from build123d import *

# Parameters (mm, degrees)
SKETCH2_R           = 28.55
BOSS_EXTRUDE1_DEPTH = 12.6
SKETCH3_R           = 21
CUT_EXTRUDE1_DEPTH  = 3
SKETCH4_R           = 15.5
CUT_EXTRUDE2_DEPTH  = 24
SKETCH5_R           = 2.2
CUT_EXTRUDE3_DEPTH  = 24


with BuildPart() as part:
    # Sketch2 → Boss-Extrude1 (new body)
    with BuildSketch(Plane(origin=(0, 0, 0), x_dir=(1, 0, 0), z_dir=(0, 1, 0))):
        with Locations(Location((0, 0, 0), (0, 0, 270))):
            Circle(SKETCH2_R)
    extrude(amount=BOSS_EXTRUDE1_DEPTH)

    # Sketch3 → Cut-Extrude1 (cut)
    with BuildSketch(Plane.XZ):
        with Locations(Location((0, 0, 0), (0, 0, 270))):
            Circle(SKETCH3_R)
    extrude(amount=-CUT_EXTRUDE1_DEPTH, mode=Mode.SUBTRACT)

    # Sketch4 → Cut-Extrude2 (cut)
    with BuildSketch(Plane.XZ.offset(-3)):
        with Locations(Location((0, 0, 0), (0, 0, 270))):
            Circle(SKETCH4_R)
    extrude(amount=-CUT_EXTRUDE2_DEPTH, mode=Mode.SUBTRACT)

    # Sketch5 → Cut-Extrude3 (cut)
    with BuildSketch(Plane(origin=(0, 0, 0), x_dir=(-1, 0, 0), z_dir=(0, -1, 0))):
        with Locations(Location((-24.775, 0, 0), (0, 0, 90))):
            Circle(SKETCH5_R)
    cut_extrude3 = extrude(amount=-CUT_EXTRUDE3_DEPTH, mode=Mode.SUBTRACT)

    # Mirror1: Cut-Extrude3 across plane
    add(cut_extrude3.mirror(Plane(origin=(0, 0, 0), x_dir=(0, 0, 1), z_dir=(1, 0, 0))), mode=Mode.SUBTRACT)


solid = part.part
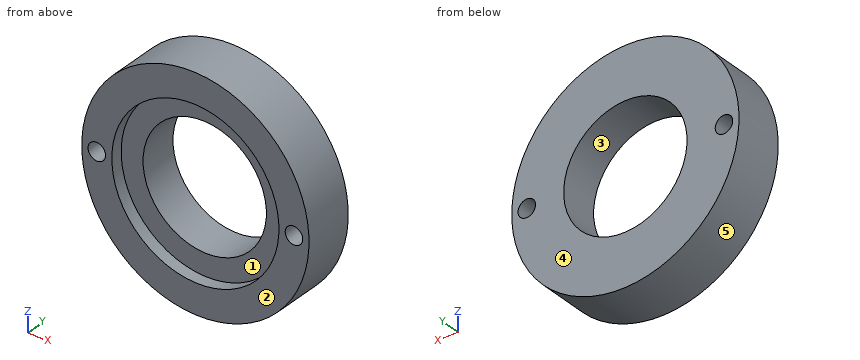
Build history of the part. All positions in model axes, mm. Face numbers are marked on the shaded views. A direction names the side the tool comes from. Coordinates: 2 decimals unless noted, no trailing zeros. Order: outer loops, then holes, each group sorted by start corner. A loop starts at its lowest first (then second) coordinate and runs counter-clockwise, first axis right, second up. Notation, with made-up numbers: (-31, 80) - (14, 80) arc R37 cw to (14, 117) - close; hole circle Ø6 at (39, 61.25). An arc over 180 degrees is marked (long way). Write item = value, one per line. Start each with the question number.
1) Two-plate mould, pull along X, no slides. Class the marked faces 3, 4 and 5: pulls with the +X half, pulls with the -X half, needs draft (parallel to the pull), parting line crosses it, or undercut.
2) Saw through at C-C on z = -14. Write the cut outline in (x, y), then the cut area to 3 significant figures.
3) Saw through at B-B on x = 0. Write the cut outline in (y, z).
4) Flat gauge pins, fed straight in: pin 1 Ø12.5 at (x, z) = (-4.5, -8) entering from -Y; pin 2 Ø1 at (y, z) = (7, -1) entering from -X; pin 3 Ø1 at (x, z) = (17, -3.5) entering from -Y; pin 4 Ø2 at (x, y) = (-13, 7.5) entering from +Z. Where does each tip first touch, or does it go through?
5) 3-axis set-ups, long thin cutter, end or side, ignore diameter. For the marked faces 1 and 2: which of +Z, -Z, +X, -X, +Y, -Y reach the whole face in a straight line?
6) Saw through at D-D on x = -18. Write the cut outline in (y, z), then the cut area to 3 significant figures.
7) Saw through at A-A on z = 0. Write the cut outline in (x, y) (3 decimals), then the cut area to 3 significant figures.
8) Wall check: line 1 along X through (y, z) = (9, 0) (3 decimals); line 2 along X through (y, z) = (1.3, 0) (3 decimals); line 3 along Z through (x, y) = (-0.5, 3.25). Give the ranges that are in metal, low to high. Write a range as from..to.
From the geometry:
q1.face_3 = undercut
q1.face_4 = needs draft
q1.face_5 = parting line crosses it
q2.outline = (-24.88, 0) - (-15.65, 0) - (-15.65, 3) - (-6.65, 3) - (-6.65, 12.6) - (-24.88, 12.6) - close; (6.65, 3) - (15.65, 3) - (15.65, 0) - (24.88, 0) - (24.88, 12.6) - (6.65, 12.6) - close
q2.area = 405 mm^2
q3.outline = (0, -28.55) - (12.6, -28.55) - (12.6, -15.5) - (3, -15.5) - (3, -21) - (0, -21) - close; (0, 21) - (3, 21) - (3, 15.5) - (12.6, 15.5) - (12.6, 28.55) - (0, 28.55) - close
q4.pin_1 = through
q4.pin_2 = -28.55
q4.pin_3 = 3
q4.pin_4 = 25.91
q5.face_1 = -Y
q5.face_2 = +Z, -Z, +X, -X, -Y
q6.outline = (0, -22.16) - (12.6, -22.16) - (12.6, 22.16) - (0, 22.16) - (0, 10.82) - (3, 10.82) - (3, -10.82) - (0, -10.82) - close
q6.area = 494 mm^2
q7.outline = (-28.55, 0) - (-26.975, 0) - (-26.975, 12.6) - (-28.55, 12.6) - close; (-22.575, 0) - (-21, 0) - (-21, 3) - (-15.5, 3) - (-15.5, 12.6) - (-22.575, 12.6) - close; (15.5, 3) - (21, 3) - (21, 0) - (22.575, 0) - (22.575, 12.6) - (15.5, 12.6) - close; (26.975, 0) - (28.55, 0) - (28.55, 12.6) - (26.975, 12.6) - close
q7.area = 185 mm^2
q8.line_1 = -28.55..-26.975, -22.575..-15.5, 15.5..22.575, 26.975..28.55
q8.line_2 = -28.55..-26.975, -22.575..-21, 21..22.575, 26.975..28.55
q8.line_3 = -28.55..-15.49, 15.49..28.55
